```python
from build123d import *

# Parameters (mm, degrees)
SKETCH1_W           = 76.2
SKETCH1_H           = 76.2
SKETCH1_W_2         = 69.85
SKETCH1_H_2         = 69.85
BOSS_EXTRUDE1_DEPTH = 132
SKETCH2_R           = 15.875
SKETCH2_R_2         = 7.9375
CUT_EXTRUDE1_DEPTH  = 158.105219519


with BuildPart() as part:
    # Sketch1 → Boss-Extrude1 (new, symmetric)
    with BuildSketch(Plane.XY):
        Rectangle(SKETCH1_W, SKETCH1_H)
        Rectangle(SKETCH1_W_2, SKETCH1_H_2, mode=Mode.SUBTRACT)
    extrude(amount=BOSS_EXTRUDE1_DEPTH, both=True)

    # Sketch2 → Cut-Extrude1 (cut, through all)
    with BuildSketch(Plane.ZY.offset(38.1)):
        Circle(SKETCH2_R)
        with Locations((-49.4109375, 0)):
            Circle(SKETCH2_R_2)
        with Locations((49.4109375, 0)):
            Circle(SKETCH2_R_2)
    extrude(amount=-CUT_EXTRUDE1_DEPTH, mode=Mode.SUBTRACT)


solid = part.part
```
Geometry: final body of the model. Coordinates: model frame, mm. A direction names the side the tool comes from. Give positions to 0.01 mm unless a question says otherwise; leave off trailing zeros. Loops run counter-clockwise (first coordinate to the right, second up) from the corner with the lowest first, then second, coordinate; pieces in that order, holes last. Notation, with made-up numbers: (59, 58.25) -> (102, 58.25) arc R33 cw to (102, 90.25) -> close; hole circle Ø5 at (-23, -31). An arc over 180 degrees is marked (long way). Return JSON: item names as keys, results as strings.
Item 1: Mould query, pull axis Z, two halves, no side actions, for faces 1 (the flat face through (-3, -37, -132)), 2 (the cylindrical face through (36.49, 0.35, 41.48)), 3 (the flat face through (0, -34.925, 2)). Classes: released by +Z, released by -Z, zero draft, split by the parting line, or undercut.
Filled in:
{"face 1": "released by -Z", "face 2": "undercut", "face 3": "zero draft"}
Item 2: Access query for faces 4 (the flat face through (-34.925, -16, 2)), 5 (the flat face through (-1, 38.1, 2)). Directions: +Z, -Z, +X, -X, +Y, -Y. A direction counts if a zero-diameter tool reaches every point of the face in a straight line with its end or side. Return the directions, or none.
Filled in:
{"face 4": "+Z, -Z", "face 5": "+Z, -Z, +X, -X, +Y"}
Item 3: Pin query (flat end, axial travel): P1, Ø9.5, axis at y = 0, z = -49.41, coming from the -X side. Return the tip coordinate at first contact, or that it passes through.
Filled in:
{"P1": "through"}
Item 4: Section A-A, the plane z = 0. Output: boundary loops of the cut face in (x, y) (3 decimals), plus the area to 3 significant figures.
Filled in:
{"outline": "(-38.1, -38.1) -> (38.1, -38.1) -> (38.1, -15.875) -> (34.925, -15.875) -> (34.925, -34.925) -> (-34.925, -34.925) -> (-34.925, -15.875) -> (-38.1, -15.875) -> close; (-38.1, 15.875) -> (-34.925, 15.875) -> (-34.925, 34.925) -> (34.925, 34.925) -> (34.925, 15.875) -> (38.1, 15.875) -> (38.1, 38.1) -> (-38.1, 38.1) -> close", "area": "726 mm^2"}
Item 5: Section D-D, the plane z = -39. Output: boundary loops of the cut face in (x, y) (3 decimals).
Filled in:
{"outline": "(-38.1, -38.1) -> (38.1, -38.1) -> (38.1, 38.1) -> (-38.1, 38.1) -> close; hole (-34.925, -34.925) -> (34.925, -34.925) -> (34.925, 34.925) -> (-34.925, 34.925) -> close"}
Item 6: Section C-C, the plane y = 0. Count the separate pieces of the cut face and the enclosed holes in it, plus the area to 3 significant figures.
Filled in:
{"separate pieces": "8", "enclosed holes": "0", "area": "1,270 mm^2"}
Item 7: Section B-B, the plane x = 5.5. Output: boundary loops of the cut face in (y, z) (3 decimals).
Filled in:
{"outline": "(-38.1, -132) -> (-34.925, -132) -> (-34.925, 132) -> (-38.1, 132) -> close; (34.925, -132) -> (38.1, -132) -> (38.1, 132) -> (34.925, 132) -> close"}
Item 8: Line query: line 1 (Y direction, x = -3.5, z = 49.5) (3 decimals). Output: solid intervals per line, ascending.
Filled in:
{"line 1": "-38.1 to -34.925, 34.925 to 38.1"}
